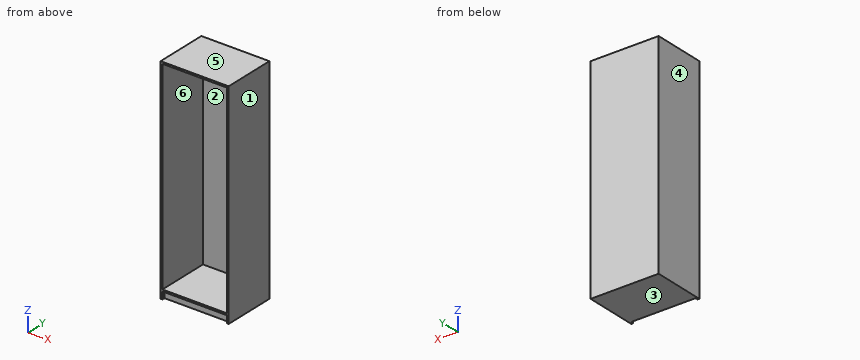
from build123d import *

# Parameters (mm, degrees)
F0_W     = 750
F0_H     = 2360
F1_DEPTH = 580
F2_W     = 710
F2_H     = 2240
F4_DEPTH = 577
F5_W     = 710
F5_H     = 80
F6_DEPTH = 30


with BuildPart() as f1:
    # F0 (on Front) → F1 (new body)
    with BuildSketch(Plane.XZ):
        with Locations((0, 1180)):
            Rectangle(F0_W, F0_H)
    extrude(amount=F1_DEPTH)

    # F2 (on face) → F4 (cut, through all)
    with BuildSketch(Plane.XZ.offset(580)):
        with Locations((0, 1220)):
            Rectangle(F2_W, F2_H)
    extrude(amount=-F4_DEPTH, mode=Mode.SUBTRACT)

    # F5 (on face) → F6 (cut)
    with BuildSketch(Plane.XZ.offset(580)):
        with Locations((0, 40)):
            Rectangle(F5_W, F5_H)
    extrude(amount=-F6_DEPTH, mode=Mode.SUBTRACT)


solid = f1.part
The model under review builds one solid part; all positions refer to its coordinate system, in mm. Face numbers are marked on the shaded views. A direction names the side the tool comes from. Round coordinates to 2 decimals unless told otherwise and drop trailing zeros. Loops run counter-clockwise (first coordinate to the right, second up) from the corner with the lowest first, then second, coordinate; pieces in that order, holes last. Notation, with made-up numbers: (14.25, -33) -> (51.25, -33) arc R36 ccw to (51.25, 4) -> close; hole circle Ø3 at (54.25, 75.25). An arc over 180 degrees is marked (long way). One line per question, with ' | ' between items. Start each with the question number.
Item 1: Add section B-B, the plane z = 617. Write out the cut boundary in (x, y).
Item 2: Machinability: for the marked faces 1 and 2, which of the approach directions +Z, -Z, +X, -X, +Y, -Y give a long, thin tool a straight path to every point of the face, cutting with its end or side? Answer none if there is none.
Item 3: Add section C-C, the plane x = 154.5. Write out the cut boundary in (y, z), then the cut area to 3 significant figures.
Item 4: Add section A-A, the plane y = -328.5. Write out the cut boundary in (x, z), then the cut area to 3 significant figures.
Item 5: For pin 1 (4 mm diameter, centred on x = 249.5, z = 862, fed in from -Y), flat-tipped, find the tip position at first contact; note if it passes through.
Item 6: Draft analysis for pull direction Z (two halves, no side actions). For the marked faces 3, 4, 5 and 6, state which applies: +Z half, -Z half, draft (parallel to the pull), parting line (faces both ways), or undercut.
Item 7: Wall thickness on line 1 along Z through (x, y) = (-144.5, -68); line 2 along X through (y, z) = (-396.5, 1977.5); line 3 along Y through (x, z) = (249.5, 827.5): over which ranges is each line inside the solid? List them lowest first. Write a range as [from, to].
Return value:
1) outline: (-375, -580) -> (-355, -580) -> (-355, -3) -> (355, -3) -> (355, -580) -> (375, -580) -> (375, 0) -> (-375, 0) -> close
2) face 1: +Z, -Z, +X, +Y, -Y | face 2: -Y
3) outline: (-580, 80) -> (-550, 80) -> (-550, 0) -> (0, 0) -> (0, 2360) -> (-580, 2360) -> (-580, 2340) -> (-3, 2340) -> (-3, 100) -> (-580, 100) -> close | area: 73,900 mm2
4) outline: (-375, 0) -> (375, 0) -> (375, 2360) -> (-375, 2360) -> close; hole (-355, 100) -> (355, 100) -> (355, 2340) -> (-355, 2340) -> close | area: 180,000 mm2
5) pin 1: stops at y = -3
6) face 3: -Z half | face 4: draft | face 5: +Z half | face 6: undercut
7) line 1: z = [0, 100], [2340, 2360] | line 2: x = [-375, -355], [355, 375] | line 3: y = [-3, 0]
